Input: part model. Units: mm. Frame: model coordinates. Face numbers are marked on the shaded views. A direction names the side the tool comes from. Round coordinates to 2 decimals unless told otherwise and drop trailing zeros. Order: outer loops, then holes, each group sorted by start corner. A loop starts at its lowest first (then second) coordinate and runs counter-clockwise, first axis right, second up.
Item 1: First-contact query: pin 1 (4 mm diameter, centred on x = 4.5, z = 9.5, fed in from +Y); pin 2 (2.5 mm diameter, centred on x = 0, z = 26.55, fed in from -Y); pin 3 (10.5 mm diameter, centred on y = -17, z = -5, fed in from -X); pin 4 (9 mm diameter, centred on x = -4, z = 0, fed in from +Y). Flat tips, straight axial feed; report the tip coordinate or a pass-through.
Item 2: Line query: L1, parallel to Z at x = 4, y = -1.5; L2, parallel to Y at x = -9, z = 17.5; L3, parallel to Y at x = -6.75, z = 3. Output: solid intervals per line, ascending.
Item 3: Cut plane C-C on y = -22. Output: boundary loops of the cut face in (x, z) (3 decimals), then the cut area to 3 significant figures.
Item 4: Reachability of the marked faces 1, 2 and 3 from +Z, -Z, +X, -X, +Y, -Y: full face, straight path, thin tool, end or side. Return the list, or none.
Item 5: Mould query, pull axis Y, two halves, no side actions, for the marked faces 4, 5, 6 and 7. Classes: released by +Y, released by -Y, zero draft, split by the parting line, or undercut.
Item 6: Cut plane A-A on z = -26.55. Output: boundary loops of the cut face in (x, y), then the cut area to 3 significant figures.
Item 7: Cut plane D-D on x = 6.75. Output: boundary loops of the cut face in (y, z).
Item 8: Cut plane B-B on x = 0. Give the number of separate pieces and of enclosed holes in the cut face, then the cut area to 3 significant figures.
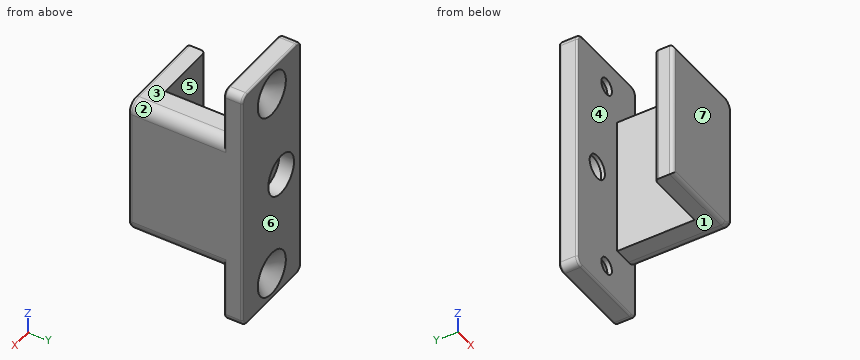
```python
from build123d import *

# Parameters (mm, degrees)
SKETCH1_W           = 25
SKETCH1_H           = 68.1
BOSS_EXTRUDE1_DEPTH = 31.05
CUT_EXTRUDE1_REACH  = 54.426
SKETCH2_W           = 15
SKETCH2_H           = 26.05
SKETCH3_W           = 17
SKETCH3_H           = 21.05
CUT_EXTRUDE2_DEPTH  = 25
FILLET5_R           = 3.175
FILLET2_R           = 1
FILLET6_R           = 2
FILLET3_R           = 0.5


with BuildPart() as part:
    # Sketch1 → Boss-Extrude1 (new body)
    with BuildSketch(Plane(origin=(0, 0, 0), x_dir=(1, 0, 0), z_dir=(0, 1, 0))):
        Rectangle(SKETCH1_W, SKETCH1_H)
    extrude(amount=-BOSS_EXTRUDE1_DEPTH)

    # Sketch2 → Cut-Extrude1 (cut, up to next)
    with BuildSketch(Plane(origin=(12.5, 0, 0), x_dir=(0, 0, -1), z_dir=(1, 0, 0)), mode=Mode.PRIVATE) as cut_extrude1_sk1:
        with Locations((-26.55, -18.025)):
            Rectangle(SKETCH2_W, SKETCH2_H)
    cut_extrude1_tool1 = extrude(cut_extrude1_sk1.sketch, amount=-CUT_EXTRUDE1_REACH, mode=Mode.PRIVATE) & part.part
    # Sketch2 → Cut-Extrude1 (cut, up to next)
    with BuildSketch(Plane(origin=(12.5, 0, 0), x_dir=(0, 0, -1), z_dir=(1, 0, 0)), mode=Mode.PRIVATE) as cut_extrude1_sk2:
        with Locations((26.55, -18.025)):
            Rectangle(SKETCH2_W, SKETCH2_H)
    cut_extrude1_tool2 = extrude(cut_extrude1_sk2.sketch, amount=-CUT_EXTRUDE1_REACH, mode=Mode.PRIVATE) & part.part
    add(cut_extrude1_tool1.solids().sort_by_distance((12.5, -18.025, 26.55))[0], mode=Mode.SUBTRACT)
    add(cut_extrude1_tool2.solids().sort_by_distance((12.5, -18.025, -26.55))[0], mode=Mode.SUBTRACT)

    # Sketch3 → Cut-Extrude2 (cut, symmetric)
    with BuildSketch(Plane.XY):
        with Locations((-4, -15.525)):
            Rectangle(SKETCH3_W, SKETCH3_H)
    extrude(amount=CUT_EXTRUDE2_DEPTH, both=True, mode=Mode.SUBTRACT)

    # Sketch5 → Cut-Revolve1 (revolve, cut)
    with BuildSketch(Plane(origin=(0, 0, 0), x_dir=(0, 0, -1), z_dir=(1, 0, 0)), mode=Mode.PRIVATE) as cut_revolve1_sk:
        Polygon((-32.55, 0), (-28.8, -3.75), (-28.8, -5), (-26.55, -5), (-26.55, 0), align=None)
    cut_revolve1 = revolve(cut_revolve1_sk.sketch.rotate(Axis((0, -5, 26.55), (0, 1, 0)), 180), axis=Axis((0, -5, 26.55), (0, 1, 0)), mode=Mode.SUBTRACT)

    # Mirror1: Cut-Revolve1 across plane
    add(cut_revolve1.mirror(Plane.XY), mode=Mode.SUBTRACT)

    # Sketch6 → Cut-Revolve2 (revolve, cut)
    with BuildSketch(Plane.XY, mode=Mode.PRIVATE) as cut_revolve2_sk:
        Polygon((-4, 0), (-4, -5), (-0.75, -5), (-0.75, -4), (1.5, -4), (1.5, 0), align=None)
    revolve(cut_revolve2_sk.sketch.rotate(Axis((-4, 0, 0), (0, -1, 0)), 180), axis=Axis((-4, 0, 0), (0, -1, 0)), mode=Mode.SUBTRACT)

    # Fillet5
    fillet5_edges = [part.edges().sort_by_distance(p)[0] for p in [
        (12.5, -18.025, 19.05),
        (12.5, -18.025, -19.05),
    ]]
    fillet(fillet5_edges, radius=FILLET5_R)

    # Fillet2
    fillet2_edges = [part.edges().sort_by_distance(p)[0] for p in [
        (-12.5, -31.05, 0),
        (-1.5875, -31.05, 19.05),
        (-1.5875, -31.05, -19.05),
        (-12.5, -26.05, 0),
        (12.5, -31.05, 0),
        (11.57006403, -31.05, -18.12006403),
        (11.57006403, -31.05, 18.12006403),
    ]]
    fillet(fillet2_edges, radius=FILLET2_R)

    # Fillet6
    fillet6_edges = [part.edges().sort_by_distance(p)[0] for p in [
        (12.5, -2.5, -34.05),
        (-12.5, -2.5, -34.05),
        (-12.5, -2.5, 34.05),
        (12.5, -2.5, 34.05),
    ]]
    fillet(fillet6_edges, radius=FILLET6_R)

    # Fillet3
    fillet3_edges = [part.edges().sort_by_distance(p)[0] for p in [
        (0, -5, 34.05),
        (0, 0, 34.05),
        (12.5, 0, 0),
        (0, 0, -34.05),
        (-12.5, 0, 0),
        (-11.914213562, 0, -33.464213562),
        (11.914213562, 0, -33.464213562),
        (-11.914213562, 0, 33.464213562),
        (11.914213562, 0, 33.464213562),
        (12.5, -5, -23.9625),
        (-12.5, -5, 0),
        (0, -5, -34.05),
        (-11.914213562, -5, -33.464213562),
        (11.914213562, -5, -33.464213562),
        (-11.914213562, -5, 33.464213562),
        (11.914213562, -5, 33.464213562),
        (12.5, -5, 23.9625),
    ]]
    fillet(fillet3_edges, radius=FILLET3_R)


solid = part.part
```
From the geometry:
1. pin 1: stops at y = 0
1. pin 2: passes through
1. pin 3: stops at x = 4.5
1. pin 4: stops at y = -4
2. L1: z = -34.05 to -28.61, -24.49 to 24.49, 28.61 to 34.05
2. L2: y = -31.05 to -26.05, -5 to 0
2. L3: y = -31.05 to -26.05, -5 to -4
3. outline: (4.5, -19.05) - (9.325, -19.05) arc R3.175 ccw to (12.5, -15.875) - (12.5, 15.875) arc R3.175 ccw to (9.325, 19.05) - (4.5, 19.05) - close
3. area: 300 mm2
4. face 1: -Z, +X, -X, -Y
4. face 2: +Z, +X, -Y
4. face 3: +Z, +X, -X, -Y
5. face 4: undercut
5. face 5: undercut
5. face 6: released by +Y
5. face 7: released by -Y
6. outline: (-12.5, -4.5) arc R0.5 ccw to (-12, -5) - (-2.25, -5) - (-2.25, -3.75) - (-6, 0) - (-12, 0) arc R0.5 ccw to (-12.5, -0.5) - close; (2.25, -5) - (12, -5) arc R0.5 ccw to (12.5, -4.5) - (12.5, -0.5) arc R0.5 ccw to (12, 0) - (6, 0) - (2.25, -3.75) - close
6. area: 88.2 mm2
7. outline: (-31.05, -18.05) arc R1 ccw to (-30.05, -19.05) - (-5, -19.05) - (-5, -33.55) arc R0.5 ccw to (-4.5, -34.05) - (-0.5, -34.05) arc R0.5 ccw to (0, -33.55) - (0, 33.55) arc R0.5 ccw to (-0.5, 34.05) - (-4.5, 34.05) arc R0.5 ccw to (-5, 33.55) - (-5, 19.05) - (-30.05, 19.05) arc R1 ccw to (-31.05, 18.05) - close
8. separate pieces: 4
8. enclosed holes: 0
8. area: 427 mm2
